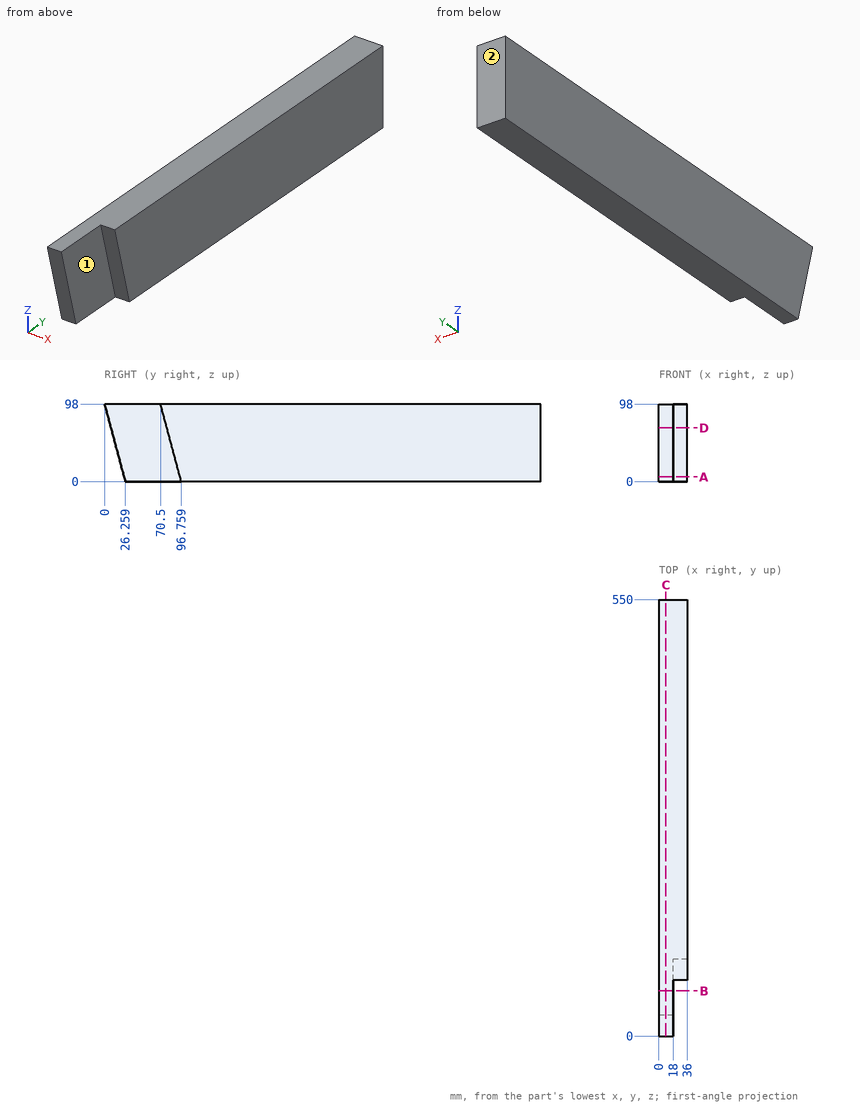
Study the drawing (mm; zero at the part's minimum x, y, z) and answer. A direction names the side the tool comes from. Coordinates: 2 decimals unless noted, no trailing zeros. Loops run counter-clockwise (first coordinate to the right, second up) from the corner with the lowest first, then second, coordinate; pieces in that order, holes last. Notation, with made-up numbers: (13, 13) -> (52, 13) arc R14 cw to (52, 26) -> close; hole circle Ø6 at (86, 78). An arc over 180 degrees is marked (long way). Write item = value, one per line. Start each with the question number.
1) The part is cut by section A-A, the plane z = 6. Determine the outline of the cut face in (x, y), plus the area to 3 significant figures.
2) The part is cut by section C-C, the plane x = 9. Determine the outline of the cut face in (y, z), plus the area to 3 significant figures.
3) Find the intervals of material crossed by L1, parallel to Y at x = 22.5, z = 57.5; L2, parallel to Y at x = 30, z = 86.5, in increasing order. Write a range as from..to.
4) The part is cut by section D-D, the plane z = 68. Determine the outline of the cut face in (x, y).
5) For the marked faces 1 and 2, determine the directions among +Z, -Z, +X, -X, +Y, -Y from which every point of the face is accessible in a straight line to the end or side of a thin tool.
6) Given P1, Ø1.5, axis at x = 13.5, z = 28.5, coming from the -Y side; P2, Ø6, axis at x = 27.5, z = 84.5, coming from the -Y side, each flat-ended and moving along its own axis, determine where each tip first touches the part or whether it passes through.
7) The part is cut by section B-B, the plane y = 57. Determine the outline of the cut face in (x, z), plus the area to 3 significant figures.
Result:
q1.outline = (0, 24.65) -> (18, 24.65) -> (18, 95.15) -> (36, 95.15) -> (36, 550) -> (0, 550) -> close
q1.area = 17,600 mm²
q2.outline = (0, 98) -> (26.26, 0) -> (550, 0) -> (550, 98) -> close
q2.area = 52,600 mm²
q3.L1 = 81.35..550
q3.L2 = 73.58..550
q4.outline = (0, 8.04) -> (18, 8.04) -> (18, 78.54) -> (36, 78.54) -> (36, 550) -> (0, 550) -> close
q5.face_1 = -Z, +X, -Y
q5.face_2 = +Z, -Z, +X, -X, +Y
q6.P1 = 18.42
q6.P2 = 73.31
q7.outline = (0, 0) -> (18, 0) -> (18, 98) -> (0, 98) -> close
q7.area = 1,760 mm²
